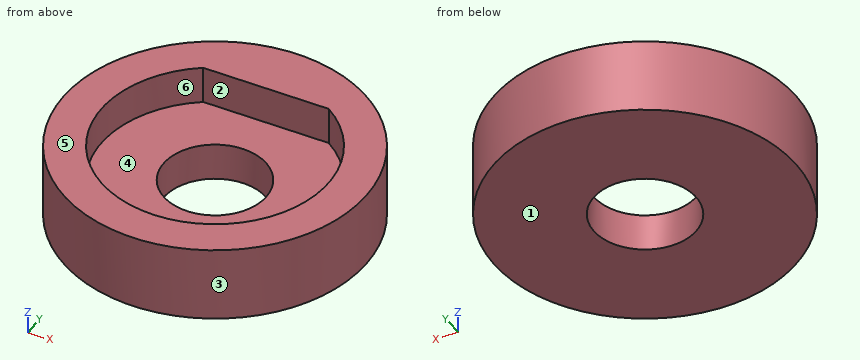
from build123d import *

# Parameters (mm, degrees)
F0_R     = 6.35
F0_R_2   = 2.15265
F1_DEPTH = 1.5875
F2_R     = 6.35
F3_DEPTH = 1.5875


with BuildPart() as f1:
    # F0 (on Top) → F1 (new body)
    with BuildSketch(Plane.XY):
        Circle(F0_R)
        Circle(F0_R_2, mode=Mode.SUBTRACT)
    extrude(amount=F1_DEPTH)

    # F2 (on face) → F3 (join)
    with BuildSketch(Plane.XY.offset(1.5875)):
        Circle(F2_R)
        with BuildLine():
            ThreePointArc((2.632571, 3.96875), (0, -4.7625), (-2.632571, 3.96875))
            Line((-2.632571, 3.96875), (2.632571, 3.96875))
        make_face(mode=Mode.SUBTRACT)
    extrude(amount=F3_DEPTH)


solid = f1.part
Geometry check sheet. Reference: the model listing, model coordinates, mm. Face numbers are marked on the shaded views. A direction names the side the tool comes from. Round coordinates to 2 decimals unless told otherwise and drop trailing zeros. Order: outer loops, then holes, each group sorted by start corner. A loop starts at its lowest first (then second) coordinate and runs counter-clockwise, first axis right, second up. Notation, with made-up numbers: M 73,-5.75 L 98,-5.75 A30 cw 98,25.25 Z; hole C 47,52.25 d7. An arc over 180 degrees is marked long. Answer in a Markdown table with one row per item. Add a question column.
Item 1: Material ranges on L1, parallel to Y at x = 0, z = 2.55; L2, parallel to Y at x = 0, z = 0.8; L3, parallel to Z at x = -0.5, y = -3.75, recorded low to high. Write a range as [from, to].
Item 2: Sectioned sample at C-C, the plane z = 0.4. Enter the section's corners in (x, y).
Item 3: Sectioned sample at D-D, the plane y = -4. Enter the section's corners in (x, z) (1 decimal), plus the area to 3 significant figures.
Item 4: Depth check by flat-ended pin: pin 1 Ø7 at (x, y) = (-0.5, -1) entering from +Z; pin 2 Ø1 at (y, z) = (3, 1) entering from -X. Enter the tip coordinate at first touch or a pass-through.
Item 5: Set-up check for the marked faces 5 and 6: record each of +Z, -Z, +X, -X, +Y, -Y from which the full face is reachable in a straight line by a thin tool's end or side.
Item 6: Draft check along X on the marked faces 1, 2, 3 and 4. Enter one of: released by +X, released by -X, zero draft, split by the parting line, or undercut.
Filled in:
| question | item | result |
|---|---|---|
| 1 | L1 | y = [-6.35, -4.76], [3.97, 6.35] |
| 1 | L2 | y = [-6.35, -2.15], [2.15, 6.35] |
| 1 | L3 | z = [0, 1.59] |
| 2 | outline | C 0,0 d12.7; hole C 0,0 d4.31 |
| 3 | outline | M -4.9,0 L 4.9,0 L 4.9,3.2 L 2.6,3.2 L 2.6,1.6 L -2.6,1.6 L -2.6,3.2 L -4.9,3.2 Z |
| 3 | area | 23.1 mm² |
| 4 | pin 1 | stops at z = 1.59 |
| 4 | pin 2 | stops at x = -5.84 |
| 5 | face 5 | +Z, +X, -X, +Y, -Y |
| 5 | face 6 | +Z |
| 6 | face 1 | zero draft |
| 6 | face 2 | undercut |
| 6 | face 3 | split by the parting line |
| 6 | face 4 | undercut |
